```python
from build123d import *

# Parameters (mm, degrees)
SKETCH1_W               = 60
SKETCH1_H               = 20
BOSS_EXTRUDE1_DEPTH     = 2
SKETCH2_R               = 2.5
BOSS_EXTRUDE2_DEPTH     = 4
SKETCH3_R               = 1
BOSS_EXTRUDE3_DEPTH     = 4
CUT_EXTRUDE1_DEPTH      = 10
CUT_EXTRUDE1_DEPTH_BACK = 10
SKETCH4_R               = 3.75
SKETCH5_W               = 60
SKETCH5_H               = 20
BOSS_EXTRUDE4_DEPTH     = 2
SKETCH6_R               = 2.5
BOSS_EXTRUDE5_DEPTH     = 4


with BuildPart() as part:
    # Sketch1 → Boss-Extrude1 (new body)
    with BuildSketch(Plane(origin=(0, 0, 0), x_dir=(1, 0, 0), z_dir=(0, 1, 0))):
        Rectangle(SKETCH1_W, SKETCH1_H)
    extrude(amount=BOSS_EXTRUDE1_DEPTH)

    # Sketch2 → Boss-Extrude2 (add)
    with BuildSketch(Plane(origin=(0, 2, 0), x_dir=(1, 0, 0), z_dir=(0, 1, 0))):
        with Locations(Location((-14, 0, 0), (0, 0, 270))):
            Circle(SKETCH2_R)
    extrude(amount=BOSS_EXTRUDE2_DEPTH)

    # Sketch3 → Boss-Extrude3 (add)
    with BuildSketch(Plane(origin=(0, 2, 0), x_dir=(1, 0, 0), z_dir=(0, 1, 0))):
        with Locations(Location((15.75, 0, 0), (0, 0, 270))):
            Circle(SKETCH3_R)
    extrude(amount=BOSS_EXTRUDE3_DEPTH)

    # Sketch4 → Cut-Extrude1 (cut, two sides: drawn at the far end of the back side and taken through both)
    with BuildSketch(Plane(origin=(0, 2, 0), x_dir=(1, 0, 0), z_dir=(0, 1, 0)).offset(-CUT_EXTRUDE1_DEPTH_BACK)):
        with Locations(Location((15.75, 0, 0), (0, 0, 270))):
            Circle(SKETCH4_R)
    extrude(amount=CUT_EXTRUDE1_DEPTH + CUT_EXTRUDE1_DEPTH_BACK, mode=Mode.SUBTRACT)

    # Sketch5 → Boss-Extrude4 (add)
    with BuildSketch(Plane(origin=(0, 2, 0), x_dir=(1, 0, 0), z_dir=(0, 1, 0))):
        with Locations((0, 20)):
            Rectangle(SKETCH5_W, SKETCH5_H)
    extrude(amount=-BOSS_EXTRUDE4_DEPTH)

    # Sketch6 → Boss-Extrude5 (add)
    with BuildSketch(Plane(origin=(0, 2, 0), x_dir=(1, 0, 0), z_dir=(0, 1, 0))):
        with Locations(Location((-6, 25, 0), (0, 0, 270))):
            Circle(SKETCH6_R)
        with Locations(Location((6, 25, 0), (0, 0, 270))):
            Circle(SKETCH6_R)
    extrude(amount=BOSS_EXTRUDE5_DEPTH)


solid = part.part
```
Here's how the part is built. I have some questions about the finished solid (model axes, mm). A direction names the side the tool comes from. Coordinates: 2 decimals unless noted, no trailing zeros. Write each loop counter-clockwise with the first axis right and the second up, starting at its lowest first coordinate (ties: lowest second). Pieces come first, ordered by that corner, then holes. Notation, with made-up numbers: M 49.25,78.25 L 75.25,78.25 A35 cw 75.25,113.25 Z; hole C -37,11.25 d3. An arc over 180 degrees is marked long. Answer as CSV lines item,"result". Start each with the question number.
Q1. I need wall thicknesses on probe 1 along X at (y, z) = (0.55, 0); probe 2 along Z at (x, y) = (15.75, 1.2); probe 3 along Y at (x, z) = (26, -27.5). Which ranges of each line are inside material? Lowest first, please. Write a range as [from, to].
Q2. Suppose I cut it at C-C, the plane y = 2.8. List the corners of the cut face in (x, z) for me.
Q3. For faces 1 (the flat face through (0, 0, -10)), 2 (the cylindrical face through (-5.9, 4, -27.5)), which set-ups out of +Z, -Z, +X, -X, +Y, -Y let a thin tool reach every point of the face, with its end or its side?
Q4. Suppose I cut it at B-B, the plane x = -14. List the corners of the cut face in (y, z) for me.
Q5. Will these pins go through, and if not, where does the flat tip stop? pin 1 Ø1.5 at (y, z) = (3.5, -25) entering from +X; pin 2 Ø4.5 at (x, z) = (15.75, 0) entering from -Y.
Q6. Suppose I cut it at D-D, the plane z = -25. List the corners of the cut face in (x, y) for me, then the cut area to 3 significant figures.
Q7. Suppose I cut it at A-A, the plane z = 0. List the corners of the cut face in (x, y) for me, then the cut area to 3 significant figures.
Q8. If we mould it in two halves opening along X, with no side actions, what happens to faces 3 (the flat face through (30, 1, -10)), 4 (the flat face through (0, 1, 10)), 5 (the cylindrical face through (12.09, 0.99, -0.81)), 6 (the cylindrical face through (7.69, 3.97, -26.84))? For each: pulls with the +X half, pulls with the -X half, needs draft (parallel to the pull), parting line crosses it, or undercut.
Entries:
1,probe 1,"x = [-30, 12], [19.5, 30]"
1,probe 2,"z = [-30, -3.75], [3.75, 10]"
1,probe 3,"y = [0, 2]"
2,outline,"C -14,0 d5; C -6,-25 d5; C 6,-25 d5"
3,face 1,"+Z, -Z, +X, -X, -Y"
3,face 2,"+Y"
4,outline,"M 0,-30 L 2,-30 L 2,-2.5 L 6,-2.5 L 6,2.5 L 2,2.5 L 2,10 L 0,10 Z"
5,pin 1,"stops at x = 8.5"
5,pin 2,"passes through"
6,outline,"M -30,0 L 30,0 L 30,2 L 8.5,2 L 8.5,6 L 3.5,6 L 3.5,2 L -3.5,2 L -3.5,6 L -8.5,6 L -8.5,2 L -30,2 Z"
6,area,"160 mm²"
7,outline,"M -30,0 L 12,0 L 12,2 L -11.5,2 L -11.5,6 L -16.5,6 L -16.5,2 L -30,2 Z; M 19.5,0 L 30,0 L 30,2 L 19.5,2 Z"
7,area,"125 mm²"
8,face 3,"pulls with the +X half"
8,face 4,"needs draft"
8,face 5,"undercut"
8,face 6,"undercut"
